```python
from build123d import *
from build123d.topology import SkipClean

# Parameters (mm, degrees)
SKETCH1_R           = 12.5
SKETCH1_R_2         = 1.75
SKETCH1_R_3         = 5.75
SKETCH1_R_4         = 7.5
SKETCH1_R_5         = 3.25
SKETCH1_W           = 10
SKETCH1_H           = 7
BOSS_EXTRUDE1_DEPTH = 10
BOSS_EXTRUDE2_START = 35
SKETCH2_R           = 3.25
SKETCH2_R_2         = 7.5
BOSS_EXTRUDE2_DEPTH = 35
SKETCH3_R           = 2.5
CUT_EXTRUDE1_DEPTH  = 35


with BuildPart() as part:
    # Sketch1 → Boss-Extrude1 (new body)
    # profile 1 of 8: a face of its own
    with BuildSketch(Plane.XY):
        with BuildLine():
            Line((-12.5, 30), (-12.5, 0))
            ThreePointArc((-12.5, 0), (0, 12.5), (12.5, 0))
            Line((12.5, 0), (12.5, 30))
            Line((12.5, 30), (-12.5, 30))
        make_face()
    # profile 2 of 8: a face of its own
    with BuildSketch(Plane.XY):
        Circle(SKETCH1_R)
        with Locations((-5.656854249, -5.656854249)):
            Circle(SKETCH1_R_2, mode=Mode.SUBTRACT)
        with Locations((5.656854249, -5.656854249)):
            Circle(SKETCH1_R_2, mode=Mode.SUBTRACT)
        with Locations((5.656854249, 5.656854249)):
            Circle(SKETCH1_R_2, mode=Mode.SUBTRACT)
        with Locations((-5.656854249, 5.656854249)):
            Circle(SKETCH1_R_2, mode=Mode.SUBTRACT)
        Circle(SKETCH1_R_3, mode=Mode.SUBTRACT)
    # profile 3 of 8: a face of its own
    with BuildSketch(Plane.XY):
        with Locations((-75.25, 0)):
            Circle(SKETCH1_R_4)
        with Locations((-75.25, 0)):
            Circle(SKETCH1_R_5, mode=Mode.SUBTRACT)
    # profile 4 of 8: a face of its own
    with BuildSketch(Plane.XY):
        with Locations((75.25, 0)):
            Circle(SKETCH1_R_4)
        with Locations((75.25, 0)):
            Circle(SKETCH1_R_5, mode=Mode.SUBTRACT)
    # profile 5 of 8: a face of its own
    with BuildSketch(Plane.XY):
        with BuildLine():
            Line((12.5, 30), (12.5, 0))
            ThreePointArc((12.5, 0), (11.858541226, -3.952847075), (10, -7.5))
            Line((10, -7.5), (75.25, -7.5))
            ThreePointArc((75.25, -7.5), (69.946699141, 5.303300859), (82.75, 0))
            Line((82.75, 0), (82.75, 23))
            Line((82.75, 23), (82.75, 30))
            Line((82.75, 30), (12.5, 30))
        make_face()
    # profile 6 of 8: a face of its own
    with BuildSketch(Plane.XY):
        with BuildLine():
            ThreePointArc((-10, -7.5), (-11.858541226, -3.952847075), (-12.5, 0))
            Line((-12.5, 0), (-12.5, 30))
            Line((-12.5, 30), (-82.75, 30))
            Line((-82.75, 30), (-82.75, 23))
            Line((-82.75, 23), (-82.75, 0))
            ThreePointArc((-82.75, 0), (-75.25, 7.5), (-67.75, 0))
            ThreePointArc((-67.75, 0), (-69.946699141, -5.303300859), (-75.25, -7.5))
            Line((-75.25, -7.5), (-10, -7.5))
        make_face()
    # profile 7 of 8: a face of its own
    with BuildSketch(Plane.XY):
        with Locations((-87.75, 26.5)):
            Rectangle(SKETCH1_W, SKETCH1_H)
    # profile 8 of 8: a face of its own
    with BuildSketch(Plane.XY):
        with Locations((87.75, 26.5)):
            Rectangle(SKETCH1_W, SKETCH1_H)
    extrude(amount=BOSS_EXTRUDE1_DEPTH)

    # Sketch2 → Boss-Extrude2 (add)
    # profile 1 of 4: a face of its own
    with SkipClean():  # the faces are left unmerged after this step: merging them gives an invalid solid
        with BuildSketch(Plane(origin=(0, 0, 0), x_dir=(-1, 0, 0), z_dir=(0, 0, -1)).offset(BOSS_EXTRUDE2_START)):
            with BuildLine():
                Line((-82.75, 23), (-82.75, 0))
                ThreePointArc((-82.75, 0), (-75.25, -7.5), (-67.75, 0))
                Line((-67.75, 0), (-67.75, 30))
                Line((-67.75, 30), (-92.75, 30))
                Line((-92.75, 30), (-92.75, 23))
                Line((-92.75, 23), (-82.75, 23))
            make_face()
            with Locations((-75.25, 0)):
                Circle(SKETCH2_R, mode=Mode.SUBTRACT)
        # profile 2 of 4: a face of its own
        with BuildSketch(Plane(origin=(0, 0, 0), x_dir=(-1, 0, 0), z_dir=(0, 0, -1)).offset(BOSS_EXTRUDE2_START)):
            with BuildLine():
                Line((92.75, 30), (67.75, 30))
                Line((67.75, 30), (67.75, 0))
                ThreePointArc((67.75, 0), (75.25, -7.5), (82.75, 0))
                Line((82.75, 0), (82.75, 23))
                Line((82.75, 23), (92.75, 23))
                Line((92.75, 23), (92.75, 30))
            make_face()
            with Locations((75.25, 0)):
                Circle(SKETCH2_R, mode=Mode.SUBTRACT)
        # profile 3 of 4: a face of its own
        with BuildSketch(Plane(origin=(0, 0, 0), x_dir=(-1, 0, 0), z_dir=(0, 0, -1)).offset(BOSS_EXTRUDE2_START)):
            with Locations(Location((-25, 12.5, 0), (0, 0, 180))):
                Circle(SKETCH2_R_2)
        # profile 4 of 4: a face of its own
        with BuildSketch(Plane(origin=(0, 0, 0), x_dir=(-1, 0, 0), z_dir=(0, 0, -1)).offset(BOSS_EXTRUDE2_START)):
            with Locations(Location((25, 12.5, 0), (0, 0, 180))):
                Circle(SKETCH2_R_2)
        extrude(amount=-BOSS_EXTRUDE2_DEPTH)

    # Sketch3 → Cut-Extrude1 (cut)
    with SkipClean():  # the faces are left unmerged after this step: merging them gives an invalid solid
        with BuildSketch(Plane(origin=(0, 30, 0), x_dir=(1, 0, 0), z_dir=(0, 1, 0))):
            with Locations(Location((-87.75, 30, 0), (0, 0, 180))):
                Circle(SKETCH3_R)
            with Locations(Location((-87.75, -5, 0), (0, 0, 180))):
                Circle(SKETCH3_R)
            with Locations(Location((87.75, 30, 0), (0, 0, 180))):
                Circle(SKETCH3_R)
            with Locations(Location((87.75, -5, 0), (0, 0, 180))):
                Circle(SKETCH3_R)
        extrude(amount=-CUT_EXTRUDE1_DEPTH, mode=Mode.SUBTRACT)


solid = part.part
```
Verification items for the finished model (mm, model axes). A direction names the side the tool comes from. Coordinates: 2 decimals unless noted, no trailing zeros. Loops run counter-clockwise (first coordinate to the right, second up) from the corner with the lowest first, then second, coordinate; pieces in that order, holes last. Notation, with made-up numbers: (44.25, -12) -> (88.25, -12) arc R27 ccw to (88.25, 26) -> close; hole circle Ø6 at (-8.75, 85). An arc over 180 degrees is marked (long way). Answer in a Markdown table with one row per item.
1) Access from +Z, -Z, +X, -X, +Y, -Y to the whole of each face (thin tool, end or side, straight path). Record for faces 5 (the face through (7.273, 4.987, 4.93)), 6 (the face through (82.75, 12, -13)), 7 (the face through (-25, 12, -35)), 8 (the face through (-67.75, 15, -18)), 9 (the face through (-32.493, 12.17, -17.745)).
The answers:
| item | result |
|---|---|
| face 5 | +Z, -Z |
| face 6 | +Z, -Z, +X, -Y |
| face 7 | -Z, +X, -X, +Y, -Y |
| face 8 | -Z, +Y, -Y |
| face 9 | -Z |
2) Section check B-B (x = -87.75). Record the cut outline in (y, z).
The answers:
| item | result |
|---|---|
| outline | (23, -35) -> (30, -35) -> (30, -32.5) -> (23, -32.5) -> close; (23, -27.5) -> (30, -27.5) -> (30, 2.5) -> (23, 2.5) -> close; (23, 7.5) -> (30, 7.5) -> (30, 10) -> (23, 10) -> close |
3) Depth check by flat-ended pin: P1, Ø6, axis at x = -87.75, z = -30, coming from the -Y side; P2, Ø6, axis at x = -75.25, y = 0, coming from the +Z side; P3, Ø7, axis at y = 7, z = -9.5, coming from the +X side; P4, Ø1, axis at y = -5, z = 0, coming from the -X side. Enter the tip coordinate at first touch or a pass-through.
The answers:
| item | result |
|---|---|
| P1 | stops at y = 23 |
| P2 | passes through |
| P3 | stops at x = 82.75 |
| P4 | stops at x = -81.25 |
4) Section check C-C (y = 17). Record the cut outline in (x, z).
The answers:
| item | result |
|---|---|
| outline | (-82.75, -35) -> (-67.75, -35) -> (-67.75, 0) -> (-31, 0) -> (-31, -35) -> (-19, -35) -> (-19, 0) -> (19, 0) -> (19, -35) -> (31, -35) -> (31, 0) -> (67.75, 0) -> (67.75, -35) -> (82.75, -35) -> (82.75, 10) -> (-82.75, 10) -> close |
5) Draft check along Z on faces 1 (the face through (-85.252, 26.549, 5.11)), 2 (the face through (7.273, -6.327, 4.93)), 3 (the face through (78, 16, -35)), 4 (the face through (90.248, 26.549, 5.11)). Enter one of: released by +Z, released by -Z, zero draft, split by the parting line, or undercut.
The answers:
| item | result |
|---|---|
| face 1 | undercut |
| face 2 | zero draft |
| face 3 | released by -Z |
| face 4 | undercut |
6) Section check D-D (z = 5). Give the number of separate pieces and of enclosed holes in the cut face, and give its area (3 significant figures).
The answers:
| item | result |
|---|---|
| separate pieces | 3 |
| enclosed holes | 7 |
| area | 6,110 mm2 |
7) Scan lines: line 1 along X through (y, z) = (13, -8.5); line 2 along X through (y, z) = (0, -22); line 3 along Z through (x, y) = (-87.75, 27.5). Record each from-to range of solid material in increasing order. Write a range as from..to.
The answers:
| item | result |
|---|---|
| line 1 | x = -82.75..-67.75, -32.48..-17.52, 17.52..32.48, 67.75..82.75 |
| line 2 | x = -82.75..-78.5, -72..-67.75, 67.75..72, 78.5..82.75 |
| line 3 | z = -35..-32.5, -27.5..2.5, 7.5..10 |
8) Section check A-A (z = -4.5). Record the cut outline in (x, y).
The answers:
| item | result |
|---|---|
| outline | (-92.75, 23) -> (-82.75, 23) -> (-82.75, 0) arc R7.5 ccw to (-67.75, 0) -> (-67.75, 30) -> (-92.75, 30) -> close; circle Ø15 at (-25, 12.5); circle Ø15 at (25, 12.5); (67.75, 0) arc R7.5 ccw to (82.75, 0) -> (82.75, 23) -> (92.75, 23) -> (92.75, 30) -> (67.75, 30) -> close; hole circle Ø6.5 at (-75.25, 0); hole circle Ø6.5 at (75.25, 0) |
